```python
from build123d import *

# Parameters (mm, degrees)
F0_W     = 900
F0_H     = 89
F1_DEPTH = 38
F3_D     = 20
F5_D     = 1


with BuildPart() as f1:
    # F0 (on Front) → F1 (new body)
    with BuildSketch(Plane.XZ):
        Rectangle(F0_W, F0_H)
    extrude(amount=F1_DEPTH)

    # F3 (through all)
    with Locations(Plane.XZ.offset(38)):
        with Locations((-350, 0)):
            Hole(F3_D / 2)

    # F5 (through all)
    with Locations(Plane.XZ.offset(38)):
        with Locations((-150, 0)):
            Hole(F5_D / 2)


solid = f1.part
```
Verification items for the finished model (mm, model axes). Coordinates: 2 decimals unless noted, no trailing zeros. Order: outer loops, then holes, each group sorted by start corner. A loop starts at its lowest first (then second) coordinate and runs counter-clockwise, first axis right, second up. Notation, with made-up numbers: (88.25, 0.25) -> (120.25, 0.25) arc R26 ccw to (120.25, 33.25) -> close; hole circle Ø5 at (11, -18). An arc over 180 degrees is marked (long way). Answer as CSV lines item,"result". Start each with the question number.
1) Material ranges on L1, parallel to Z at x = -350, y = -27; L2, parallel to Z at x = -150, y = -15; L3, parallel to X at y = -30.5, z = -5.5, recorded low to high. Write a range as [from, to].
2) Release check for a two-part mould opening along Z. For faces 1 (the face through (-6, -19, 44.5)), 2 (the face through (-340, -19, 0)), 3 (the face through (-6, -38, 1)) record: released by +Z, released by -Z, zero draft, split by the parting line, or undercut.
3) Cross-section at A-A, the plane x = -350. Record the boundary of the cut face in (y, z).
4) Gauge pin test, flat end, axial feed: pin 1 Ø4 at (x, z) = (-31, 35.5) entering from +Y. Record the tip position at first contact, or that the pin passes through.
Conclusion:
1,L1,"z = [-44.5, -10], [10, 44.5]"
1,L2,"z = [-44.5, -0.5], [0.5, 44.5]"
1,L3,"x = [-450, -358.35], [-341.65, 450]"
2,face 1,"released by +Z"
2,face 2,"undercut"
2,face 3,"zero draft"
3,outline,"(-38, -44.5) -> (0, -44.5) -> (0, -10) -> (-38, -10) -> close; (-38, 10) -> (0, 10) -> (0, 44.5) -> (-38, 44.5) -> close"
4,pin 1,"stops at y = 0"
